Input: part model. Units: mm. Frame: model coordinates. A direction names the side the tool comes from. Round coordinates to 2 decimals unless told otherwise and drop trailing zeros. Order: outer loops, then holes, each group sorted by start corner. A loop starts at its lowest first (then second) coordinate and runs counter-clockwise, first axis right, second up. Notation, with made-up numbers: (23.25, 53.25) -> (71.25, 53.25) arc R21 ccw to (71.25, 75.25) -> close; hole circle Ø7 at (44, 42.5). An arc over 180 degrees is marked (long way). Use a Markdown table: item, result.
Autodesk Fusion 360 part; units mm, degrees
sketch "Sketch1" plane through (0, 0, 0) normal (0, 1, 0) x (1, 0, 0)
  circle A0 centre (0, 0) radius 25
  line L0 (0, 0) -> (0, -72.8192) construction
  line L1 (0, -72.8192) -> (0, 0) construction
  line L2 (0, -45) -> (-4.9923, -44.7222)
  line L3 (-4.9923, -44.7222) -> (-4.3266, -38.7593)
  line L4 (-14.7457, -42.5154) -> (-12.7796, -36.8467)
  line L5 (-23.771, -38.2091) -> (-20.6016, -33.1146)
  line L6 (-31.6224, -32.016) -> (-27.4061, -27.7472)
  line L7 (-37.9122, -24.2417) -> (-32.8573, -21.0095)
  line L8 (-42.3298, -15.2704) -> (-36.6859, -13.2344)
  line L9 (-44.6571, -5.545) -> (-38.7028, -4.8057)
  line L10 (0, 0) -> (-2.7735, -24.8457) construction
  line L11 (-4.3266, -38.7593) -> (-4.9923, -44.7222) construction
  line L12 (0, 0) -> (-8.1921, -23.6197) construction
  line L13 (-12.7796, -36.8467) -> (-14.7457, -42.5154) construction
  line L14 (0, 0) -> (-13.2061, -21.2273) construction
  line L15 (-20.6016, -33.1146) -> (-23.771, -38.2091) construction
  line L16 (0, 0) -> (-17.568, -17.7866) construction
  line L17 (-27.4061, -27.7472) -> (-31.6224, -32.016) construction
  line L18 (0, 0) -> (-21.0624, -13.4676) construction
  line L19 (-32.8573, -21.0095) -> (-37.9122, -24.2417) construction
  line L20 (0, 0) -> (-23.5166, -8.4836) construction
  line L21 (-36.6859, -13.2344) -> (-42.3298, -15.2704) construction
  line L22 (0, 0) -> (-24.8095, -3.0805) construction
  line L23 (-38.7028, -4.8057) -> (-44.6571, -5.545) construction
  arc A1 (-23.771, -38.2091) -> (-14.7457, -42.5154) centre (0, 0) ccw
  arc A2 (-37.9122, -24.2417) -> (-31.6224, -32.016) centre (0, 0) ccw
  arc A3 (-36.6859, -13.2344) -> (-32.8573, -21.0095) centre (0, 0) ccw
  arc A4 (-27.4061, -27.7472) -> (-20.6016, -33.1146) centre (0, 0) ccw
  line L24 (-44.7805, 4.4388) -> (-38.8098, 3.847) construction
  line L25 (0, 0) -> (-24.8781, 2.466) construction
  line L26 (-38.8098, 3.847) -> (-44.7805, 4.4388) construction
  line L27 (-44.7805, 4.4388) -> (-38.8098, 3.847)
  arc A5 (-44.6571, -5.545) -> (-42.3298, -15.2704) centre (0, 0) ccw
  line L28 (0, -45) -> (4.9923, -44.7222)
  line L29 (0, 0) -> (4.9923, -44.7222) construction
  line L30 (4.9923, -44.7222) -> (4.3266, -38.7593)
  line L31 (0.0235, -39) -> (0, -45) construction
  line L32 (0.0235, -39) -> (0, -45)
  arc A6 (-12.7796, -36.8467) -> (-4.3266, -38.7593) centre (0, 0) ccw
  line L33 (0, 0) -> (67, 0) construction
  line L34 (0, 0) -> (0, 30) construction
  line L35 (65.5098, -16.7592) -> (65.5098, -18.6386)
  line L36 (0, 0) -> (14.7457, -42.5154) construction
  line L37 (0, 0) -> (23.771, -38.2091) construction
  line L38 (0, 0) -> (31.6224, -32.016) construction
  line L39 (0, 0) -> (37.9122, -24.2417) construction
  line L40 (0, 0) -> (42.3298, -15.2704) construction
  line L41 (0, 0) -> (44.6571, -5.545) construction
  line L42 (12.7796, -36.8467) -> (14.7457, -42.5154)
  line L43 (20.6016, -33.1146) -> (23.771, -38.2091)
  line L44 (27.4061, -27.7472) -> (31.6224, -32.016)
  line L45 (32.8573, -21.0095) -> (37.9122, -24.2417)
  line L46 (36.6859, -13.2344) -> (42.3298, -15.2704)
  line L47 (38.7028, -4.8057) -> (44.6571, -5.545)
  arc A7 (-4.9923, -44.7222) -> (4.9923, -44.7222) centre (0, 0) ccw
  line L48 (4.9923, -44.7222) -> (14.7457, -42.5154) construction
  arc A8 (14.7457, -42.5154) -> (23.771, -38.2091) centre (0, 0) ccw
  line L49 (23.771, -38.2091) -> (31.6224, -32.016) construction
  arc A9 (31.6224, -32.016) -> (37.9122, -24.2417) centre (0, 0) ccw
  line L50 (37.9122, -24.2417) -> (42.3298, -15.2704) construction
  arc A10 (4.3266, -38.7593) -> (12.7796, -36.8467) centre (0, 0) ccw
  line L51 (12.7796, -36.8467) -> (20.6016, -33.1146) construction
  arc A11 (20.6016, -33.1146) -> (27.4061, -27.7472) centre (0, 0) ccw
  line L52 (27.4061, -27.7472) -> (32.8573, -21.0095) construction
  arc A12 (32.8573, -21.0095) -> (36.6859, -13.2344) centre (0, 0) ccw
  line L53 (36.6859, -13.2344) -> (38.7028, -4.8057) construction
  line L54 (-38.7028, -4.8057) -> (-36.6859, -13.2344) construction
  line L55 (-32.8573, -21.0095) -> (-27.4061, -27.7472) construction
  line L56 (-20.6016, -33.1146) -> (-12.7796, -36.8467) construction
  line L57 (-4.3266, -38.7593) -> (4.3266, -38.7593) construction
  line L58 (44.9966, -0.5565) -> (44.9725, 0)
  line L59 (0, 0) -> (44.7805, 4.4388) construction
  line L60 (0, 0) -> (42.6946, 14.2188) construction
  line L61 (0, 0) -> (38.5002, 23.2967) construction
  line L62 (0, 0) -> (32.4046, 31.2241) construction
  line L63 (0, 0) -> (24.7088, 37.6095) construction
  line L64 (0, 0) -> (15.7927, 42.1377) construction
  line L65 (0, 0) -> (6.0968, 44.5851) construction
  line L66 (38.8098, 3.847) -> (44.7805, 4.4388)
  line L67 (37.0019, 12.323) -> (42.6946, 14.2188)
  line L68 (33.3668, 20.1904) -> (38.5002, 23.2967)
  line L69 (28.084, 27.0609) -> (32.4046, 31.2241)
  line L70 (21.4143, 32.5949) -> (24.7088, 37.6095)
  line L71 (13.687, 36.5194) -> (15.7927, 42.1377)
  line L72 (5.2839, 38.6404) -> (6.0968, 44.5851)
  arc A13 (42.3298, -15.2704) -> (44.6571, -5.545) centre (0, 0) ccw
  arc A14 (44.9966, -0.5565) -> (45, 0) centre (0, 0) ccw
  line L73 (44.6571, -5.545) -> (44.7805, 4.4388) construction
  arc A15 (44.7805, 4.4388) -> (42.6946, 14.2188) centre (0, 0) ccw
  line L74 (42.6946, 14.2188) -> (38.5002, 23.2967) construction
  arc A16 (38.5002, 23.2967) -> (32.4046, 31.2241) centre (0, 0) ccw
  line L75 (32.4046, 31.2241) -> (24.7088, 37.6095) construction
  arc A17 (24.7088, 37.6095) -> (15.7927, 42.1377) centre (0, 0) ccw
  line L76 (15.7927, 42.1377) -> (6.0968, 44.5851) construction
  line L77 (1.113, 44.9862) -> (-3.8847, 44.832)
  line L78 (0, 0) -> (-3.8847, 44.832) construction
  line L79 (0, 0) -> (-13.6897, 42.8671) construction
  line L80 (0, 0) -> (-22.8188, 38.7854) construction
  line L81 (0, 0) -> (-30.8209, 32.7883) construction
  line L82 (0, 0) -> (-37.3011, 25.172) construction
  line L83 (0, 0) -> (-41.9392, 16.3127) construction
  line L84 (-3.3667, 38.8544) -> (-3.8847, 44.832)
  line L85 (-11.8644, 37.1515) -> (-13.6897, 42.8671)
  line L86 (-19.7763, 33.614) -> (-22.8188, 38.7854)
  line L87 (-26.7115, 28.4165) -> (-30.8209, 32.7883)
  line L88 (-32.3276, 21.8157) -> (-37.3011, 25.172)
  line L89 (-41.9392, 16.3127) -> (-36.3473, 14.1376)
  arc A18 (6.0968, 44.5851) -> (-3.8847, 44.832) centre (0, 0) ccw
  line L90 (-3.8847, 44.832) -> (-13.6897, 42.8671) construction
  line L91 (-13.6897, 42.8671) -> (-11.8644, 37.1515) construction
  arc A19 (-13.6897, 42.8671) -> (-22.8188, 38.7854) centre (0, 0) ccw
  line L92 (-22.8188, 38.7854) -> (-30.8209, 32.7883) construction
  line L93 (-30.8209, 32.7883) -> (-26.7115, 28.4165) construction
  line L94 (-30.8209, 32.7883) -> (-26.7115, 28.4165)
  arc A20 (-30.8209, 32.7883) -> (-37.3011, 25.172) centre (0, 0) ccw
  arc A21 (-41.9392, 16.3127) -> (-44.7805, 4.4388) centre (0, 0) ccw
  line L95 (-37.3011, 25.172) -> (-41.9392, 16.3127) construction
  line L96 (-41.9392, 16.3127) -> (-36.3473, 14.1376)
  line L97 (-32.3276, 21.8157) -> (-37.3011, 25.172)
  arc A22 (38.7028, -4.8057) -> (38.8098, 3.847) centre (0, 0) ccw
  line L98 (38.8098, 3.847) -> (37.0019, 12.323) construction
  line L99 (24.7088, 37.6095) -> (21.4143, 32.5949)
  arc A23 (37.0019, 12.323) -> (33.3668, 20.1904) centre (0, 0) ccw
  line L100 (33.3668, 20.1904) -> (28.084, 27.0609) construction
  line L101 (38.5002, 23.2967) -> (33.3668, 20.1904)
  arc A24 (28.084, 27.0609) -> (21.4143, 32.5949) centre (0, 0) ccw
  line L102 (21.4143, 32.5949) -> (13.687, 36.5194) construction
  line L103 (13.687, 36.5194) -> (15.7927, 42.1377)
  arc A25 (13.687, 36.5194) -> (5.2839, 38.6404) centre (0, 0) ccw
  line L104 (5.2839, 38.6404) -> (-3.3667, 38.8544) construction
  line L105 (-3.3667, 38.8544) -> (-3.8847, 44.832)
  line L106 (-13.6897, 42.8671) -> (-11.8644, 37.1515)
  arc A26 (-3.3667, 38.8544) -> (-11.8644, 37.1515) centre (0, 0) ccw
  line L107 (-11.8644, 37.1515) -> (-19.7763, 33.614) construction
  line L108 (-22.8188, 38.7854) -> (-19.7763, 33.614)
  line L109 (-30.8209, 32.7883) -> (-26.7115, 28.4165)
  arc A27 (-19.7763, 33.614) -> (-26.7115, 28.4165) centre (0, 0) ccw
  line L110 (-26.7115, 28.4165) -> (-32.3276, 21.8157) construction
  line L111 (-37.3011, 25.172) -> (-32.3276, 21.8157)
  line L112 (-36.3473, 14.1376) -> (-41.9392, 16.3127)
  arc A28 (-32.3276, 21.8157) -> (-36.3473, 14.1376) centre (0, 0) ccw
  arc A29 (-38.8098, 3.847) -> (-38.7028, -4.8057) centre (0, 0) ccw
  line L113 (-38.8098, 3.847) -> (-36.3473, 14.1376) construction
  line L114 (-41.9392, 16.3127) -> (-36.3473, 14.1376)
  line L115 (-32.3276, 21.8157) -> (-36.3473, 14.1376)
  dimension "d1" = 90
  dimension "d2" = 78
  dimension "d3" = 50
  dimension "d4" = 5
  dimension "d5" = 10
  dimension "d6" = 10
  dimension "d7" = 10
  dimension "d8" = 10
  dimension "d9" = 10
  dimension "d10" = 10
  dimension "d13" = 12.739
  dimension "d14" = 5
  dimension "d15" = 10
  dimension "d16" = 10
  dimension "d17" = 10
  dimension "d18" = 10
  dimension "d19" = 10
  dimension "d20" = 10
  dimension "d21" = 5
  dimension "d22" = 5
  dimension "d23" = 10
  dimension "d24" = 10
  dimension "d25" = 10
  dimension "d26" = 10
  dimension "d27" = 10
  dimension "d28" = 10
  dimension "d29" = 5
  dimension "d30" = 5
  dimension "d31" = 10
  dimension "d32" = 10
  dimension "d33" = 10
  dimension "d34" = 10
  dimension "d35" = 10
extrude "Extrude1" add sketch "Sketch1" along normal mid plane 10 contours L2 L3 L4 L5 L6 L7 L8 L9 A1 A2 A3 A4 L27 A5 L28 L30 A6 L42 L43 L44 L45 L46 L47 A8 A9 A10 A11 A12 L66 L67 L68 L69 L70 L71 L72 A13 A15 A16 A17 L77 L84 L85 L86 L87 L88 L89 A18 A19 L94 A20 A21 L96 L97 A22 L99 A23 L101 A24 L103 A25 L105 L106 A26 L108 L109 A27 L111 L112 A29 L114 L115
1) Cut plane C-C on z = 35.5. Return loops of the section in (x, y), and give its area (3 significant figures).
Answer key:
| item | result |
|---|---|
| outline | (-22.09, -5) -> (22.09, -5) -> (22.09, 5) -> (-22.09, 5) -> close |
| area | 442 mm^2 |
2) Cut plane B-B on x = -17. Return loops of the section in (y, z).
Answer key:
| item | result |
|---|---|
| outline | (-5, -41.67) -> (5, -41.67) -> (5, -18.33) -> (-5, -18.33) -> close; (-5, 18.33) -> (5, 18.33) -> (5, 41.67) -> (-5, 41.67) -> close |
3) Set-up query: faces 1 (the face through (39.81, -0.07, -13.26)), 2 (the face through (35.03, -0.07, 28.25)), 3 (the face through (22.164, -0.07, 35.626)). Return all of +Z, -Z, +X, -X, +Y, -Y with unobstructed straight access to the full face (end or side cutting, diameter ignored); none if empty.
Answer key:
| item | result |
|---|---|
| face 1 | +Y, -Y |
| face 2 | +Z, +X, +Y, -Y |
| face 3 | +X, +Y, -Y |
4) Contact query for flat-ended pins moving along their axis: P1, Ø5, axis at y = 2, z = -22.5, coming from the -X side; P2, Ø1.5, axis at y = 0, z = -33.5, coming from the +X side; P3, Ø1.5, axis at y = 0.5, z = -11.5, coming from the +X side. Output: stop coordinate, or through.
Answer key:
| item | result |
|---|---|
| P1 | stops at x = -37.05 |
| P2 | stops at x = 22.5 |
| P3 | stops at x = 43.7 |
5) Ray query, probe 1 along Z at (x, y) = (36, -4); probe 2 along X at (y, z) = (1.25, 0); probe 3 along Z at (x, y) = (-35.5, 1.25). Return the intervals inside material, ascending.
Answer key:
| item | result |
|---|---|
| probe 1 | z = -27 to -21.78, -15 to 15, 23.02 to 27 |
| probe 2 | x = -39 to -25, 25 to 39 |
| probe 3 | z = -27.65 to -23.96, -15.76 to 16.15, 22.7 to 27.65 |
6) Draft query along Z for faces 4 (the face through (-34.319, -0.07, -29.107)), 5 (the face through (-13.776, -0.07, 39.721)), 6 (the face through (-41.837, -0.07, -4.147)). Return one class per face: released by +Z, released by -Z, zero draft, split by the parting line, or undercut.
Answer key:
| item | result |
|---|---|
| face 4 | released by -Z |
| face 5 | released by +Z |
| face 6 | undercut |
7) Cut plane A-A on z = 0. Return loops of the section in (x, y), and give its area (3 significant figures).
Answer key:
| item | result |
|---|---|
| outline | (-39, -5) -> (-25, -5) -> (-25, 5) -> (-39, 5) -> close; (25, -5) -> (39, -5) -> (39, 5) -> (25, 5) -> close |
| area | 280 mm^2 |
